Design review of the part built by this model. Coordinates are the model's own, in mm. Face numbers are marked on the shaded views. A direction names the side the tool comes from. Give positions to 0.01 mm unless a question says otherwise; leave off trailing zeros. Write each loop counter-clockwise with the first axis right and the second up, starting at its lowest first coordinate (ties: lowest second). Pieces come first, ordered by that corner, then holes. Notation, with made-up numbers: (-25, 58) -> (-1, 58) arc R23 ccw to (-1, 91) -> close; hole circle Ø1 at (11, 5). An arc over 180 degrees is marked (long way). Answer as a JSON object with one key per item and string values.
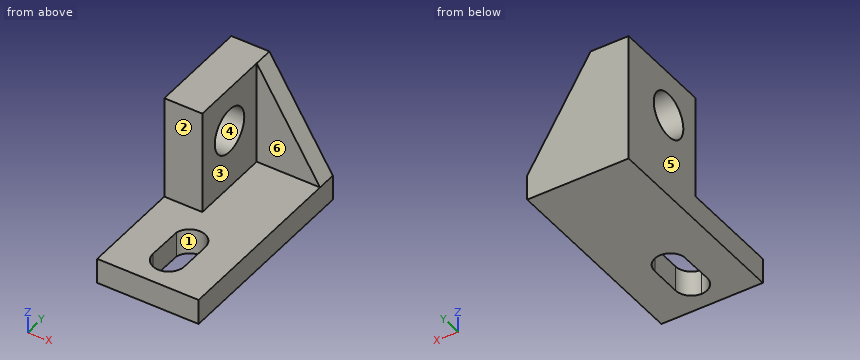
```python
from build123d import *

# Parameters (mm, degrees)
F0_W      = 101.6
F0_H      = 64.77
F1_DEPTH  = 50.8
F3_DEPTH  = 52.07
F4_R      = 11.176
F5_DEPTH  = 19.051
F6_W      = 31.75
F6_H      = 9.652
F7_DEPTH  = 52.07
F9_DEPTH  = 9.653
F11_DEPTH = 12.701


with BuildPart() as f1:
    # F0 (on Right) → F1 (new body)
    with BuildSketch(Plane.YZ):
        Rectangle(F0_W, F0_H)
    extrude(amount=F1_DEPTH)

    # F2 (on face) → F3 (cut)
    with BuildSketch(Plane.XY.offset(32.385)):
        Polygon((19.05, 0), (0, 0), (0, -50.8), (50.8, -50.8), (50.8, 50.8), (19.05, 50.8), align=None)
    extrude(amount=-F3_DEPTH, mode=Mode.SUBTRACT)

    # F4 (on face) → F5 (cut, through all)
    with BuildSketch(Plane.YZ.offset(19.05)):
        with Locations((20.574, 10.033)):
            Circle(F4_R)
    extrude(amount=-F5_DEPTH, mode=Mode.SUBTRACT)

    # F6 (on face) → F7 (join)
    with BuildSketch(Plane.XY.offset(-19.685)):
        with Locations((34.925, 45.974)):
            Rectangle(F6_W, F6_H)
    extrude(amount=F7_DEPTH)

    # F8 (on face) → F9 (cut, through all)
    with BuildSketch(Plane.XZ.offset(-41.148)):
        Polygon((50.8, 32.385), (19.05, 32.385), (50.8, -19.685), align=None)
    extrude(amount=-F9_DEPTH, mode=Mode.SUBTRACT)

    # F10 (on face) → F11 (cut, through all)
    with BuildSketch(Plane.XY.offset(-19.685)):
        with BuildLine():
            Line((17.727991, -17.53195), (17.526526, -34.960989))
            ThreePointArc((17.526526, -34.960989), (19.800156, -40.587488), (25.4, -42.926))
            ThreePointArc((25.4, -42.926), (30.967778, -40.619739), (33.274, -35.051945))
            Line((33.274, -35.051945), (33.27389, -19.345712))
            ThreePointArc((33.27389, -19.345712), (26.312481, -11.48305), (17.727991, -17.53195))
        make_face()
    extrude(amount=-F11_DEPTH, mode=Mode.SUBTRACT)


solid = f1.part
```
(1) The part is to be moulded in two halves that separate along Y. For the marked faces 4, 5 and 6, say which applies: +Y half, -Y half, draft (parallel to the pull), parting line (faces both ways), or undercut.
Here are the results:
{"face 4": "undercut", "face 5": "draft", "face 6": "-Y half"}
(2) We need section B-B, the plane y = 13. State the section outline as (x, z) points (3 decimals).
Here are the results:
{"outline": "(0, -32.385) -> (50.8, -32.385) -> (50.8, -19.685) -> (19.05, -19.685) -> (19.05, 1.815) -> (0, 1.815) -> close; (0, 18.251) -> (19.05, 18.251) -> (19.05, 32.385) -> (0, 32.385) -> close"}
(3) We need section A-A, the plane z = -21. State the section outline as (x, y) points.
Here are the results:
{"outline": "(0, -50.8) -> (50.8, -50.8) -> (50.8, 50.8) -> (0, 50.8) -> close; hole (17.53, -34.96) arc R7.87 ccw to (25.4, -42.93) arc R7.87 ccw to (33.27, -35.05) -> (33.27, -19.35) arc R7.87 ccw to (17.73, -17.53) -> close"}
(4) We need section D-D, the plane x = 14. State the section outline as (y, z) points (3 decimals).
Here are the results:
{"outline": "(-50.8, -32.385) -> (50.8, -32.385) -> (50.8, 32.385) -> (0, 32.385) -> (0, -19.685) -> (-50.8, -19.685) -> close; hole circle Ø22.352 at (20.574, 10.033)"}
(5) We need section C-C, the plane z = 16. State the section outline as (x, y) points, then the cut area to 3 significant figures.
Here are the results:
{"outline": "(0, 0) -> (19.05, 0) -> (19.05, 11.12) -> (0, 11.12) -> close; (0, 30.02) -> (19.05, 30.02) -> (19.05, 41.15) -> (29.04, 41.15) -> (29.04, 50.8) -> (0, 50.8) -> close", "area": "704 mm²"}
(6) For the marked faces 1, 2 and 3, list the 3-axis set-ups (+Z, -Z, +X, -X, +Y, -Y) from which the entire face can be reached by the end or side of a thin tool; tool diameter is ignored.
Here are the results:
{"face 1": "+Z, -Z", "face 2": "+Z, +X, -X, -Y", "face 3": "+Z, +X, -Y"}
(7) Clearance check with flat-ended pins moving along their axes: pin 1 (4 mm diameter, centred on y = -26, z = -28.5, fed in from -X); pin 2 (9.5 mm diameter, centred on x = 14, z = -2.5, fed in from -Y); pin 3 (3 mm diameter, centred on x = 28, z = 5.5, fed in from -Y); pin 4 (4 mm diameter, centred on x = 35.5, y = -21.5, fed in from +Z) (3 decimals). State where each tip first meets the part, or that it passes through.
Here are the results:
{"pin 1": "stops at x = 0", "pin 2": "stops at y = 0", "pin 3": "stops at y = 41.15", "pin 4": "stops at z = -19.685"}
(8) For line 1 along X through (y, z) = (16.5, -10); line 2 along Z through (x, y) = (36, -43) (3 decimals); line 3 along Y through (x, z) = (13, 9.5), list the stretches that pass through material, from the lowest coordinate up.
Here are the results:
{"line 1": "x = 0 to 19.05", "line 2": "z = -32.385 to -19.685", "line 3": "y = 0 to 9.41, 31.74 to 50.8"}
